The model under review builds one solid part; all positions refer to its coordinate system, in mm. Face numbers are marked on the shaded views. A direction names the side the tool comes from. Round coordinates to 2 decimals unless told otherwise and drop trailing zeros. Loops run counter-clockwise (first coordinate to the right, second up) from the corner with the lowest first, then second, coordinate; pieces in that order, holes last. Notation, with made-up numbers: M -24,84 L 6,84 A36 ccw 6,122 Z; hole C 16,-29.75 d7. An arc over 180 degrees is marked long. One line per question, with ' | ' between items.
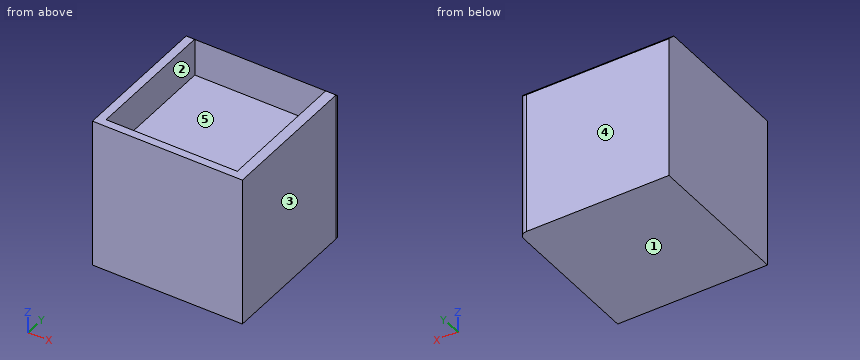
from build123d import *

# Parameters (mm, degrees)
F0_W        = 100
F0_H        = 100
F1_DEPTH    = 100
F2_W        = 87.4791443348
F2_H        = 89.9195559323
F3_DEPTH    = 25
F4_T1_DEPTH = 125.7168298797
F5_R        = 5


# Not quite as in the source:
# - a fillet or chamfer that OpenCascade refuses, or shapes differently, is made with other operations: its cross-section is extruded or revolved along the edge and cut away or added


with BuildPart() as f1:
    # F0 (on Top) → F1 (new body)
    with BuildSketch(Plane.XY):
        Rectangle(F0_W, F0_H)
    extrude(amount=F1_DEPTH)

    # F2 (on face) → F3 (cut)
    with BuildSketch(Plane.XY.offset(100)):
        with Locations((-0.6570331752, 0.2815853804)):
            Rectangle(F2_W, F2_H)
    extrude(amount=-F3_DEPTH, mode=Mode.SUBTRACT)

    # F4: chamfer of 5 on 1 edges, made by hand

    # F4_s2 → F4_t1 (cut)
    with BuildSketch(Plane.YZ.offset(-62.8584149398)):
        Polygon((50, 95), (45, 100), (50, 100), align=None)
    extrude(amount=F4_T1_DEPTH, mode=Mode.SUBTRACT)

    # F5
    f5_edges = [f1.edges().sort_by_distance(p)[0] for p in [
        (50, 50, 47.5),
    ]]
    fillet(f5_edges, radius=F5_R)


solid = f1.part
1) Add section A-A on z = 78.5. State the section outline as (x, y) points.
Output values:
outline: M -50,-50 L 50,-50 L 50,45 A5 ccw 45,50 L -50,50 Z; hole M -44.4,-44.68 L 43.08,-44.68 L 43.08,45.24 L -44.4,45.24 Z
2) Mouldability with a two-part tool opening along Y and no side actions: class the marked faces 3, 4 and 5 as +Y half, -Y half, draft (parallel to the pull), parting line (faces both ways), or undercut.
Output values:
face 3: draft | face 4: +Y half | face 5: undercut
3) Machinability: for the marked faces 1 and 2, which of the approach directions +Z, -Z, +X, -X, +Y, -Y give a long, thin tool a straight path to every point of the face, cutting with its end or side? Answer none if there is none.
Output values:
face 1: -Z, +X, -X, +Y, -Y | face 2: +Z
4) For line 1 (Y direction, x = 15, z = 93); line 2 (X direction, y = 4.5, z = 78.5); line 3 (Z direction, x = -27, y = 22.5), list the stretches that pass through material, from the lowest coordinate up.
Output values:
line 1: y = -50 to -44.68, 45.24 to 50 | line 2: x = -50 to -44.4, 43.08 to 50 | line 3: z = 0 to 75
5) Add section B-B on x = -23. State the section outline as (y, z) points, then the cut area to 3 significant figures.
Output values:
outline: M -50,0 L 50,0 L 50,95 L 45.24,99.76 L 45.24,75 L -44.68,75 L -44.68,100 L -50,100 Z | area: 7,740 mm²
6) Add section C-C on y = -32.5. State the section outline as (x, z) points, then the cut area to 3 significant figures.
Output values:
outline: M -50,0 L 50,0 L 50,100 L 43.08,100 L 43.08,75 L -44.4,75 L -44.4,100 L -50,100 Z | area: 7,810 mm²
7) Insertion check: P1, Ø8, axis at x = 38.5, y = -5, coming from the +Z side. The pin has a flat end and moves straight along its axis. Give the tip position at first contact, or say it passes through.
Output values:
P1: stops at z = 75
